Input: dimensioned drawing with shaded views. Units: mm. Origin: part minimum x, y, z. A direction names the side the tool comes from. Round coordinates to 2 decimals unless told otherwise and drop trailing zeros. Loops run counter-clockwise (first coordinate to the right, second up) from the corner with the lowest first, then second, coordinate; pieces in that order, holes last. Notation, with made-up numbers: (17.5, 73) - (53.5, 73) arc R11 ccw to (53.5, 82) - close; hole circle Ø5 at (34, 55.25). An arc over 180 degrees is marked (long way). One line per question, with ' | ' between items. Start each with the question number.
1. Access query for the marked faces 1 and 2. Directions: +Z, -Z, +X, -X, +Y, -Y. A direction counts if a zero-diameter tool reaches every point of the face in a straight line with its end or side. Return the directions, or none.
2. Cut plane B-B (z = 15.5). Return loops of the section in (x, y).
3. Ray query, line 1 (Z direction, x = 8.9, y = 5); line 2 (Y direction, x = 8.35, z = 3); line 3 (X direction, y = 12.5, z = 15). Return the intervals inside material, ascending.
4. Pin query (flat end, axial travel): pin 1 (2.5 mm diameter, centred on x = 9, y = 46, fed in from -Z); pin 2 (2 mm diameter, centred on y = 14, z = 15, fed in from -X); pin 3 (1.2 mm diameter, centred on x = 8, z = 34.5, fed in from +Y). Return the tip coordinate at first contact, or that it passes through.
5. Cut plane A-A (y = 38). Return loops of the section in (x, z).
6. Cut plane C-C (y = 5). Return loops of the section in (x, z).
7. Cut plane D-D (x = 1). Return loops of the section in (y, z), then the cut area to 3 significant figures.
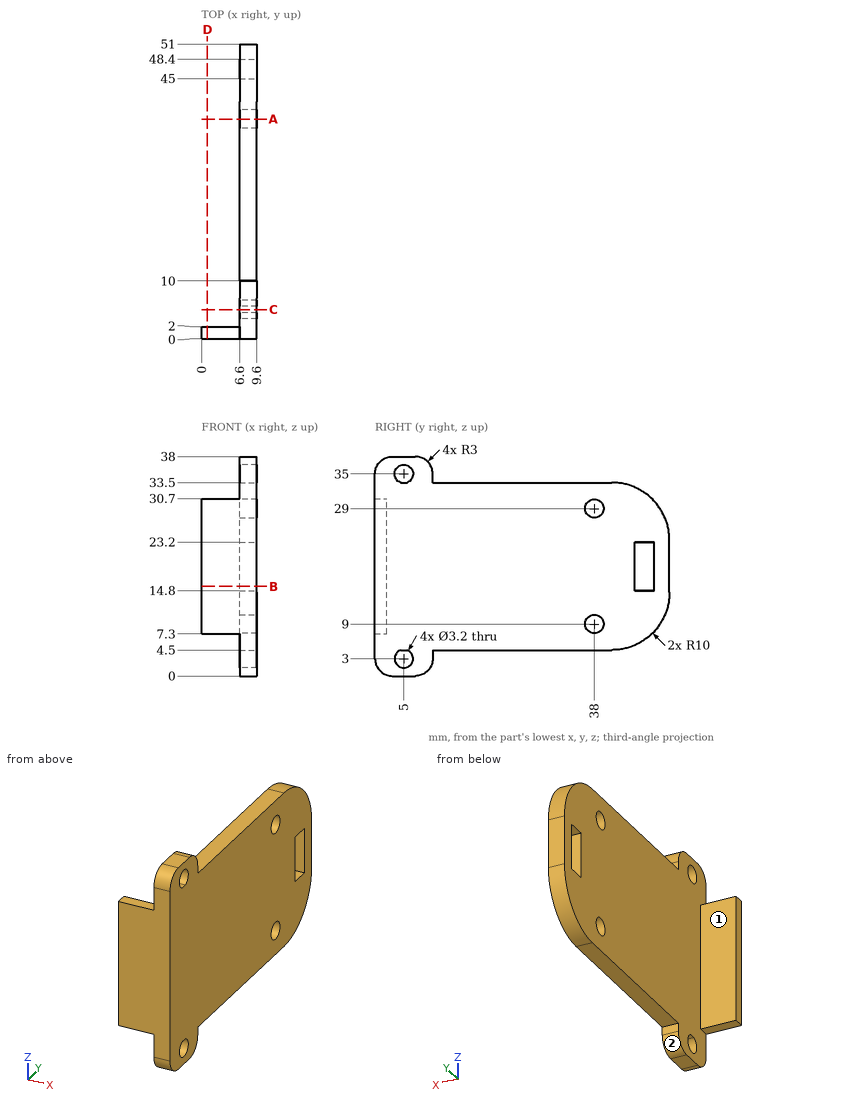
Answers follow:
1) face 1: +Z, -Z, -X, +Y | face 2: -Z, +X, -X, +Y
2) outline: (0, 0) - (9.6, 0) - (9.6, 45) - (6.6, 45) - (6.6, 2) - (0, 2) - close; (6.6, 48.4) - (9.6, 48.4) - (9.6, 51) - (6.6, 51) - close
3) line 1: z = 0 to 1.4, 4.5 to 33.5, 36.6 to 38 | line 2: y = 0 to 3.4, 6.6 to 10 | line 3: x = 6.6 to 9.6
4) pin 1: stops at z = 5.23 | pin 2: stops at x = 6.6 | pin 3: stops at y = 10
5) outline: (6.6, 4.5) - (9.6, 4.5) - (9.6, 7.4) - (6.6, 7.4) - close; (6.6, 10.6) - (9.6, 10.6) - (9.6, 27.4) - (6.6, 27.4) - close; (6.6, 30.6) - (9.6, 30.6) - (9.6, 33.5) - (6.6, 33.5) - close
6) outline: (6.6, 0) - (9.6, 0) - (9.6, 1.4) - (6.6, 1.4) - close; (6.6, 4.5) - (9.6, 4.5) - (9.6, 33.5) - (6.6, 33.5) - close; (6.6, 36.6) - (9.6, 36.6) - (9.6, 38) - (6.6, 38) - close
7) outline: (0, 7.3) - (2, 7.3) - (2, 30.7) - (0, 30.7) - close | area: 46.8 mm2
